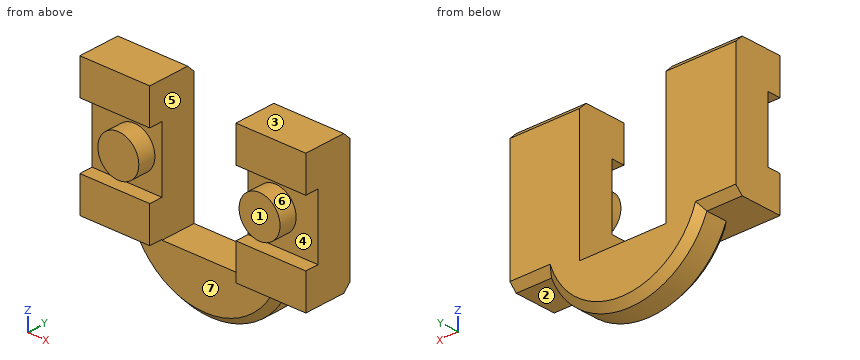
from build123d import *

# Parameters (mm, degrees)
BOSS_EXTRUDE1_DEPTH = 5
SKETCH4_W           = 9.9
SKETCH4_H           = 5
BOSS_EXTRUDE2_DEPTH = 1.9
SKETCH5_R           = 2.9
BOSS_EXTRUDE3_DEPTH = 2.5
CHAMFER1_SIZE       = 1


with BuildPart() as part:
    # Sketch3 → Boss-Extrude1 (new body)
    with BuildSketch(Plane(origin=(0, 0, 0), x_dir=(1, 0, 0), z_dir=(0, 1, 0))):
        with BuildLine():
            Line((-16, -9.5), (-6.1, -9.5))
            Line((-6.1, -9.5), (-6.1, 9.6))
            Line((-6.1, 9.6), (6.1, 9.6))
            Line((6.1, 9.6), (6.1, -9.5))
            Line((6.1, -9.5), (16, -9.5))
            Line((16, -9.5), (16, 9.5))
            Line((16, 9.5), (11, 9.5))
            ThreePointArc((11, 9.5), (0, 17), (-11, 9.5))
            Line((-11, 9.5), (-16, 9.5))
            Line((-16, 9.5), (-16, -9.5))
        make_face()
    extrude(amount=BOSS_EXTRUDE1_DEPTH)

    # Sketch4 → Boss-Extrude2 (add)
    with BuildSketch(Plane(origin=(0, 0, 0), x_dir=(1, 0, 0), z_dir=(0, 1, 0))):
        with Locations((-11.05, 7)):
            Rectangle(SKETCH4_W, SKETCH4_H)
        with Locations((-11.05, -7)):
            Rectangle(SKETCH4_W, SKETCH4_H)
        with Locations((11.05, 7)):
            Rectangle(SKETCH4_W, SKETCH4_H)
        with Locations((11.05, -7)):
            Rectangle(SKETCH4_W, SKETCH4_H)
    extrude(amount=-BOSS_EXTRUDE2_DEPTH)

    # Sketch5 → Boss-Extrude3 (add)
    with BuildSketch(Plane(origin=(0, 0, 0), x_dir=(1, 0, 0), z_dir=(0, 1, 0))):
        with Locations(Location((-10, 0, 0), (0, 0, 270))):
            Circle(SKETCH5_R)
        with Locations(Location((10, 0, 0), (0, 0, 270))):
            Circle(SKETCH5_R)
    extrude(amount=-BOSS_EXTRUDE3_DEPTH)

    # Chamfer1
    chamfer1_edges = [part.edges().sort_by_distance(p)[0] for p in [
        (0, 0, -17),
        (-11.05, 5, 9.5),
        (11.05, 5, 9.5),
        (13.5, 5, -9.5),
        (0, 5, -17),
        (-13.5, 5, -9.5),
    ]]
    chamfer(chamfer1_edges, length=CHAMFER1_SIZE)


solid = part.part
CAD build for the part. Positions are in the model's coordinates, mm. Face numbers are marked on the shaded views. A direction names the side the tool comes from. Round coordinates to 2 decimals unless told otherwise and drop trailing zeros. Loops run counter-clockwise (first coordinate to the right, second up) from the corner with the lowest first, then second, coordinate; pieces in that order, holes last.
(1) Drop flat-ended pins along their axis: pin 1 (1 mm diameter, centred on x = 9.5, y = -1, fed in from -Z); pin 2 (1 mm diameter, centred on x = 13, z = -8, fed in from -Y); pin 3 (1 mm diameter, centred on x = 8.5, y = 0.5, fed in from -Z). Give the stop position or say it passes through.
(2) Which spindle directions (+Z, -Z, +X, -X, +Y, -Y) get a long thin tool onto all of the face, cutting with end or side? Do the marked faces 5, 6 and 7. Say none if no direction does.
(3) Cut at B-B (x = 0). Give the cut face in (y, z), plus the area to 3 significant figures.
(4) Wall check: line 1 along X through (y, z) = (1.5, 6); line 2 along Z through (x, y) = (-13, 3.5); line 3 along Y through (x, z) = (7, -13). Give the ranges that are in metal, low to high.
(5) Cut at A-A (z = 0). Give the cut face in (x, y), plus the area to 3 significant figures.
(6) Cut at C-C (y = 2.5). Give the cut face in (x, z).
(7) Two-plate mould, pull along Z, no slides. Class the marked faces 1, 2, 3 and 4: +Z half, -Z half, draft (parallel to the pull), parting line (faces both ways), or undercut.
Findings below:
1. pin 1: stops at z = -9.5
1. pin 2: stops at y = -1.9
1. pin 3: stops at z = -13.55
2. face 5: +Z, +Y, -Y
2. face 6: -Y
2. face 7: -Z, +X, -X, -Y
3. outline: (0, -16) - (1, -17) - (4, -17) - (5, -16) - (5, -9.6) - (0, -9.6) - close
3. area: 36.0 mm2
4. line 1: x = -16 to -6.1, 6.1 to 16
4. line 2: z = -9.5 to 9.5
4. line 3: y = 0 to 5
5. outline: (-16, 0) - (-12.9, 0) - (-12.9, -2.5) - (-7.1, -2.5) - (-7.1, 0) - (-6.1, 0) - (-6.1, 5) - (-16, 5) - close; (6.1, 0) - (7.1, 0) - (7.1, -2.5) - (12.9, -2.5) - (12.9, 0) - (16, 0) - (16, 5) - (6.1, 5) - close
5. area: 128 mm2
6. outline: (-16, -9.5) - (-11, -9.5) arc R11.82 ccw to (11, -9.5) - (16, -9.5) - (16, 9.5) - (6.1, 9.5) - (6.1, -9.6) - (-6.1, -9.6) - (-6.1, 9.5) - (-16, 9.5) - close
7. face 1: draft
7. face 2: -Z half
7. face 3: +Z half
7. face 4: undercut
